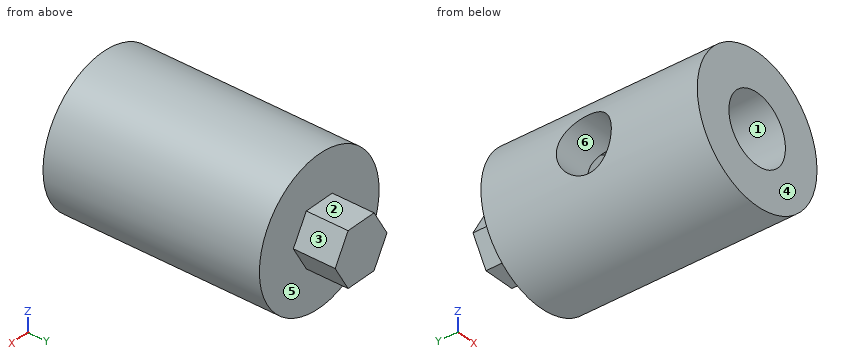
from build123d import *

# Parameters (mm, degrees)
SKETCH1_R           = 6.35
SKETCH1_R_2         = 3
BOSS_EXTRUDE1_DEPTH = 12.5
SKETCH4_R           = 2.413
CUT_EXTRUDE1_DEPTH  = 7.35
SKETCH6_R           = 6.35
BOSS_EXTRUDE4_DEPTH = 6.4925
BOSS_EXTRUDE5_DEPTH = 3.67


with BuildPart() as part:
    # Sketch1 → Boss-Extrude1 (new body)
    with BuildSketch(Plane(origin=(0, 0, 0), x_dir=(1, 0, 0), z_dir=(0, 1, 0))):
        Circle(SKETCH1_R)
        Circle(SKETCH1_R_2, mode=Mode.SUBTRACT)
    extrude(amount=BOSS_EXTRUDE1_DEPTH)

    # Sketch4 → Cut-Extrude1 (cut, through all)
    with BuildSketch(Plane(origin=(0, 0, 0), x_dir=(0, 0, -1), z_dir=(1, 0, 0))):
        with Locations((0, 9.96)):
            Circle(SKETCH4_R)
    extrude(amount=-CUT_EXTRUDE1_DEPTH, mode=Mode.SUBTRACT)

    # Sketch6 → Boss-Extrude4 (add)
    with BuildSketch(Plane(origin=(0, 12.5, 0), x_dir=(1, 0, 0), z_dir=(0, 1, 0))):
        Circle(SKETCH6_R)
    extrude(amount=BOSS_EXTRUDE4_DEPTH)

    # Sketch7 → Boss-Extrude5 (add)
    with BuildSketch(Plane(origin=(0, 18.9925, 0), x_dir=(1, 0, 0), z_dir=(0, 1, 0))):
        Polygon((-1.3748, 2.38122345), (-2.7496, 0), (-1.3748, -2.38122345), (1.3748, -2.38122345), (2.7496, 0), (1.3748, 2.38122345), align=None)
    extrude(amount=BOSS_EXTRUDE5_DEPTH)


solid = part.part
Input: part model. Units: mm. Frame: model coordinates. Face numbers are marked on the shaded views. A direction names the side the tool comes from. Coordinates: 2 decimals unless noted, no trailing zeros. Loops run counter-clockwise (first coordinate to the right, second up) from the corner with the lowest first, then second, coordinate; pieces in that order, holes last.
(1) Section B-B on x = 0. Return the cut outline in (y, z).
(2) Section D-D on y = 12.75. Return the cut outline in (x, z), then the cut area to 3 significant figures.
(3) First-contact query: pin 1 Ø0.8 at (x, y) = (0.5, 20.5) entering from +Z; pin 2 Ø4.5 at (y, z) = (9.96, 0) entering from -X; pin 3 Ø5 at (x, y) = (3, 15.5) entering from -Z. Flat tips, straight axial feed; report the tip coordinate or a pass-through.
(4) Material intervals for probe 1 along Y at (x, z) = (-5.15, 0); probe 2 along X at (y, z) = (7, 0); probe 3 along Y at (x, z) = (1, -0.25), sorted ascending.
(5) Section A-A on z = -2. Return the cut outline in (x, y).
(6) Set-up query: the marked faces 1, 2 and 3. Return all of +Z, -Z, +X, -X, +Y, -Y with unobstructed straight access to the full face (end or side cutting, diameter ignored); none if empty.
(7) Pull-direction query (Y, two-part tool) for the marked faces 4, 5 and 6; classes: released by +Y, released by -Y, zero draft, split by the parting line, or undercut.
(8) Section C-C on y = 4.75. Return the cut outline in (x, z), then the cut area to 3 significant figures.
Data:
1. outline: (0, -6.35) - (18.99, -6.35) - (18.99, -2.38) - (22.66, -2.38) - (22.66, 2.38) - (18.99, 2.38) - (18.99, 6.35) - (0, 6.35) - (0, 3) - (12.5, 3) - (12.5, -3) - (0, -3) - close
2. outline: circle Ø12.7 at (0, 0)
2. area: 127 mm2
3. pin 1: stops at z = 2.38
3. pin 2: stops at x = 1.98
3. pin 3: stops at z = -6.33
4. probe 1: y = 0 to 7.55, 12.37 to 18.99
4. probe 2: x = -6.35 to -3, 3 to 6.35
4. probe 3: y = 12.5 to 22.66
5. outline: (-6.03, 0) - (-2.24, 0) - (-2.24, 8.61) - (-6.03, 8.61) - close; (-6.03, 11.31) - (-2.24, 11.31) - (-2.24, 12.5) - (2.24, 12.5) - (2.24, 0) - (6.03, 0) - (6.03, 18.99) - (1.59, 18.99) - (1.59, 22.66) - (-1.59, 22.66) - (-1.59, 18.99) - (-6.03, 18.99) - close
6. face 1: -Y
6. face 2: +Z, +X, -X, +Y
6. face 3: +Z, +X, +Y
7. face 4: released by -Y
7. face 5: released by +Y
7. face 6: undercut
8. outline: circle Ø12.7 at (0, 0); hole circle Ø6 at (0, 0)
8. area: 98.4 mm2
